Verification items for the finished model (mm, model axes). A direction names the side the tool comes from. Give positions to 0.01 mm unless a question says otherwise; leave off trailing zeros. Write each loop counter-clockwise with the first axis right and the second up, starting at its lowest first coordinate (ties: lowest second). Pieces come first, ordered by that corner, then holes. Notation, with made-up numbers: M 61.25,6.25 L 71.25,6.25 A8 ccw 71.25,12.25 Z; hole C 60,53 d9. An arc over 180 degrees is marked long. Write item = value, one per line.
from build123d import *

# Parameters (mm, degrees)
BOSS_EXTRUDE1_DEPTH = 7.5
BOSS_EXTRUDE4_DEPTH = 3
CHAMFER7_SIZE       = 3
CHAMFER8_SIZE       = 3


with BuildPart() as part:
    # Sketch1 → Boss-Extrude1 (new body)
    with BuildSketch(Plane(origin=(0, 0, 0), x_dir=(1, 0, 0), z_dir=(0, 1, 0))):
        Polygon((-37.5, 27.5), (-27.5, 37.5), (27.5, 37.5), (37.5, 27.5), (37.5, -27.5), (27.5, -37.5), (-27.5, -37.5), (-37.5, -27.5), align=None)
    extrude(amount=BOSS_EXTRUDE1_DEPTH)

    # Sketch8 → Boss-Extrude4 (add)
    with BuildSketch(Plane(origin=(0, 0, -37.5), x_dir=(-1, 0, 0), z_dir=(0, 0, -1))):
        Polygon((-25, 3), (25, 3), (27.5, 3), (27.5, 7.5), (25, 7.5), (-25, 7.5), (-27.5, 7.5), (-27.5, 3), align=None)
    extrude(amount=BOSS_EXTRUDE4_DEPTH)

    # Chamfer7
    chamfer7_edges = [part.edges().sort_by_distance(p)[0] for p in [
        (0, 3, -40.5),
    ]]
    chamfer(chamfer7_edges, length=CHAMFER7_SIZE - 0.0001)  # a hair under: the kernel refuses the full size

    # Chamfer8
    chamfer8_edges = [part.edges().sort_by_distance(p)[0] for p in [
        (-27.5, 6.74995, -40.5),
        (27.5, 6.74995, -40.5),
    ]]
    chamfer(chamfer8_edges, length=CHAMFER8_SIZE - 0.0001)  # a hair under: the kernel refuses the full size


solid = part.part
1) Tool access check on faces 1 (the flat face through (33, 4, 32)), 2 (the flat face through (0, 1, -37.5)). Record the directions out of +Z, -Z, +X, -X, +Y, -Y that give a thin tool (end or side, any length) a straight path to the whole face; none if there is none.
From the geometry:
face_1 = +Z, +X, +Y, -Y
face_2 = -Z, +X, -X, -Y
2) Cross-section at D-D on z = 29. Record the boundary of the cut face in (x, y).
From the geometry:
outline = M -36,0 L 36,0 L 36,7.5 L -36,7.5 Z
3) Cross-section at C-C on z = -31.5. Record the boundary of the cut face in (x, y).
From the geometry:
outline = M -33.5,0 L 33.5,0 L 33.5,7.5 L -33.5,7.5 Z
4) Depth check by flat-ended pin: P1, Ø3.5, axis at x = -0.5, y = 1.5, coming from the -Z side; P2, Ø12, axis at x = 25.5, z = -14.5, coming from the -Y side. Enter the tip coordinate at first touch or a pass-through.
From the geometry:
P1 = -37.75
P2 = 0
5) Material ranges on probe 1 along Z at (x, y) = (-27, 1.25); probe 2 along Z at (x, y) = (-33, 2); probe 3 along X at (y, z) = (4.5, -30.5), recorded low to high. Write a range as from..to.
From the geometry:
probe_1 = -37.5..37.5
probe_2 = -32..32
probe_3 = -34.5..34.5
6) Cross-section at B-B on y = 2. Record the boundary of the cut face in (x, z).
From the geometry:
outline = M -37.5,-27.5 L -27.5,-37.5 L 27.5,-37.5 L 37.5,-27.5 L 37.5,27.5 L 27.5,37.5 L -27.5,37.5 L -37.5,27.5 Z
